For this review, take the finished solid that the model builds, in its own axes (mm). Face numbers are marked on the shaded views. A direction names the side the tool comes from. Give positions to 0.01 mm unless a question says otherwise; leave off trailing zeros. Loops run counter-clockwise (first coordinate to the right, second up) from the corner with the lowest first, then second, coordinate; pieces in that order, holes last. Notation, with made-up numbers: (-16, 84.5) - (24, 84.5) arc R31 cw to (24, 114.5) - close; hole circle Ø7 at (44.25, -20.75). An arc over 180 degrees is marked (long way). Answer in a Markdown table with one row per item.
```python
from build123d import *

# Parameters (mm, degrees)
BOSS_EXTRUDE1_DEPTH       = 32
BOSS_EXTRUDE2_REACH       = 59.827
SKETCH3_4_R               = 6
CUT_EXTRUDE1_DEPTH        = 24
SKETCH4_W                 = 16
SKETCH4_H                 = 9
BOSS_EXTRUDE3_DEPTH       = 32
F_6_0MM_DOWEL_HOLE1_D     = 6
F_6_0MM_DOWEL_HOLE1_DEPTH = 16
F_6_0MM_DOWEL_HOLE1_TIP   = 1.802581857


# Read off the part's stored shape, not the designer's step: CBORE for M5 Hex Head Bolt1
with BuildPart() as part:
    # Sketch1 → Boss-Extrude1 (new, symmetric)
    with BuildSketch(Plane.XY):
        Polygon((0, 36), (0, 0), (32, 0), (32, 10), (10, 10), (10, 36), align=None)
    extrude(amount=BOSS_EXTRUDE1_DEPTH, both=True)

    # Sketch3 → Boss-Extrude2 (add, up to next)
    with BuildSketch(Plane(origin=(32, 0, 0), x_dir=(0, 0, -1), z_dir=(1, 0, 0)), mode=Mode.PRIVATE) as boss_extrude2_sk1:
        with BuildLine():
            Line((14.500924593, 26.761892188), (21.509410706, 11.732145215))
            ThreePointArc((21.509410706, 11.732145215), (22.616435242, 10.469825663), (24.228334067, 10))
            Line((24.228334067, 10), (-24.228334067, 10))
            ThreePointArc((-24.228334067, 10), (-22.616435242, 10.469825663), (-21.509410706, 11.732145215))
            Line((-21.509410706, 11.732145215), (-14.500924593, 26.761892188))
            ThreePointArc((-14.500924593, 26.761892188), (0, 36), (14.500924593, 26.761892188))
        make_face()
    boss_extrude2_tool1 = extrude(boss_extrude2_sk1.sketch, amount=-BOSS_EXTRUDE2_REACH, mode=Mode.PRIVATE) - part.part
    add(boss_extrude2_tool1.solids().sort_by_distance((32, 20.8085, 0))[0])

    # Sketch3<4> → Cut-Extrude1 (cut)
    with BuildSketch(Plane(origin=(32, 0, 0), x_dir=(0, 0, -1), z_dir=(1, 0, 0))):
        with Locations((0, 20)):
            Circle(SKETCH3_4_R)
    extrude(amount=-CUT_EXTRUDE1_DEPTH, mode=Mode.SUBTRACT)

    # Sketch4 → Boss-Extrude3 (add)
    with BuildSketch(Plane(origin=(32, 0, 0), x_dir=(0, 0, -1), z_dir=(1, 0, 0))):
        with Locations((0, -4.5)):
            Rectangle(SKETCH4_W, SKETCH4_H)
    extrude(amount=-BOSS_EXTRUDE3_DEPTH)

    # Ø6.0mm Dowel Hole1
    with Locations(Plane(origin=(0, -9, 0), x_dir=(-1, 0, 0), z_dir=(0, -1, 0))):
        with Locations((-8, 0), (-24, 0)):
            Hole(F_6_0MM_DOWEL_HOLE1_D / 2, depth=F_6_0MM_DOWEL_HOLE1_DEPTH)
            with Locations((0, 0, -(F_6_0MM_DOWEL_HOLE1_DEPTH + F_6_0MM_DOWEL_HOLE1_TIP / 2))):  # 118° drill point
                Cone(0, F_6_0MM_DOWEL_HOLE1_D / 2, F_6_0MM_DOWEL_HOLE1_TIP, mode=Mode.SUBTRACT)

    # CBORE for M5 Hex Head Bolt1 outline → CBORE for M5 Hex Head Bolt1 (revolve, cut)
    with BuildSketch(Plane(origin=(20, 0, 0), x_dir=(1, 0, 0), z_dir=(0, 0, 1))):
        Polygon((0, 25.195854076), (3, 25.195854076), (3, 32), (5, 32), (5, 36.000103319), (0, 36.000103319), align=None)
    revolve(axis=Axis((20, 0, 0), (0, 1, 0)), mode=Mode.SUBTRACT)


solid = part.part
```
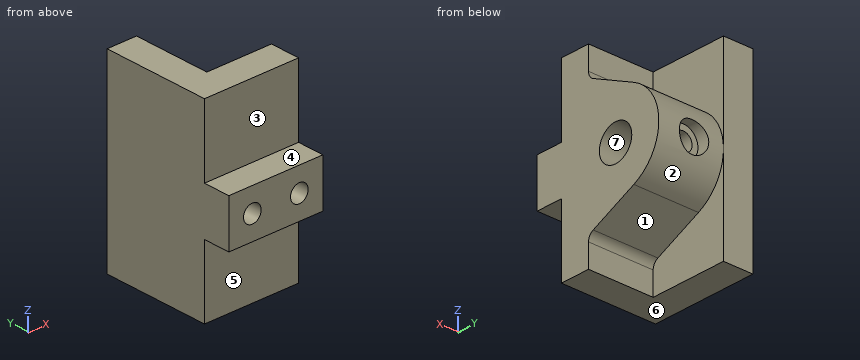
1. Wall thickness on line 1 (Z direction, x = 8, y = 2); line 2 (X direction, y = 29, z = 0); line 3 (X direction, y = 33, z = 0): over which ranges is each line inside the solid? List them lowest first. Write a range as [from, to].
Values:
| item | result |
|---|---|
| line 1 | z = [-32, -3], [3, 32] |
| line 2 | x = [0, 17], [23, 32] |
| line 3 | x = [0, 15], [25, 32] |
2. We need section A-A, the plane y = 12.5. Give the boundary of the cut face in (x, z).
Values:
| item | result |
|---|---|
| outline | (0, -32) - (10, -32) - (10, -21.15) - (32, -21.15) - (32, 21.15) - (10, 21.15) - (10, 32) - (0, 32) - close |
3. Mouldability with a two-part tool opening along Z and no side actions: class the marked faces 4, 5, 6 and 7 as released by +Z, released by -Z, zero draft, split by the parting line, or undercut.
Values:
| item | result |
|---|---|
| face 4 | released by +Z |
| face 5 | zero draft |
| face 6 | released by -Z |
| face 7 | undercut |
4. For the marked faces 1, 2 and 3, list the 3-axis set-ups (+Z, -Z, +X, -X, +Y, -Y) from which the entire face can be reached by the end or side of a thin tool; tool diameter is ignored.
Values:
| item | result |
|---|---|
| face 1 | -Z, +X, +Y |
| face 2 | +X, +Y |
| face 3 | +Z, +X, -X, -Y |
5. We need section D-D, the plane y = 29. Give the boundary of the cut face in (x, z).
Values:
| item | result |
|---|---|
| outline | (0, -32) - (10, -32) - (10, -13.23) - (32, -13.23) - (32, 13.23) - (10, 13.23) - (10, 32) - (0, 32) - close; hole circle Ø6 at (20, 0) |
6. We need section C-C, the plane x = 20. Give the boundary of the cut face in (y, z).
Values:
| item | result |
|---|---|
| outline | (-9, -8) - (0, -8) - (0, -32) - (10, -32) - (10, -24.23) arc R3 cw to (11.73, -21.51) - (26.76, -14.5) arc R16 ccw to (35.2, -5) - (32, -5) - (32, -3) - (25.2, -3) arc R6 cw (long way) to (25.2, 3) - (32, 3) - (32, 5) - (35.2, 5) arc R16 ccw to (26.76, 14.5) - (11.73, 21.51) arc R3 cw to (10, 24.23) - (10, 32) - (0, 32) - (0, 8) - (-9, 8) - close |
7. We need section B-B, the plane y = -5. Give the boundary of the cut face in (x, z), and give its area (3 significant figures).
Values:
| item | result |
|---|---|
| outline | (0, -8) - (32, -8) - (32, 8) - (0, 8) - close; hole circle Ø6 at (8, 0); hole circle Ø6 at (24, 0) |
| area | 455 mm^2 |
8. Clearance check with flat-ended pins moving along their axes: pin 1 (9.5 mm diameter, centred on x = 24, z = 0, fed in from -Y); pin 2 (6 mm diameter, centred on x = 22, y = 24, fed in from -Z); pin 3 (3.5 mm diameter, centred on x = 20, z = 0, fed in from +Y); pin 4 (6 mm diameter, centred on x = 24.5, z = 28, fed in from +Y). State where each tip first meets the part, or that it passes through.
Values:
| item | result |
|---|---|
| pin 1 | stops at y = -9 |
| pin 2 | stops at z = -17.19 |
| pin 3 | stops at y = 14.26 |
| pin 4 | stops at y = 10 |
